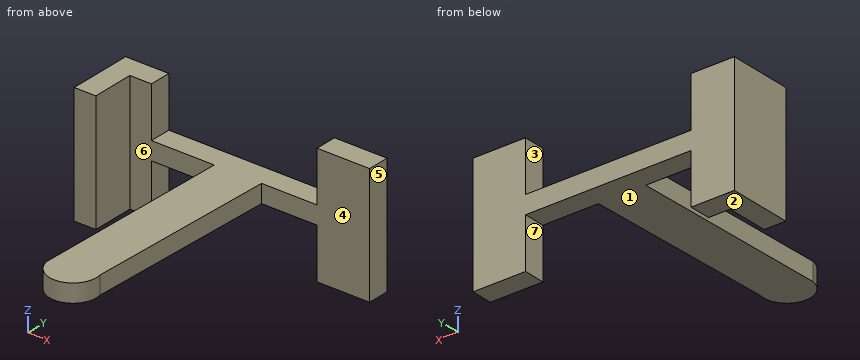
Autodesk Inventor part; units mm, degrees
ref_plane "Work Plane5" through (0, 0, 9.5) normal (0, 0, 1) x (1, 0, 0)
ref_plane "Work Plane4" through (-12.5, 22.5, 0) normal (0, 1, 0) x (1, 0, 0)
ref_plane "YZ Plane" through (0, 0, 0) normal (1, 0, 0) x (0, 1, 0)
ref_plane "Work Plane5" through (0, 0, 9.5) normal (0, 0, 1) x (1, 0, 0)
sketch "Sketch4" plane through (0, 0, 9.5) normal (0, 0, 1) x (1, 0, 0)
  arc A0 (-3.3085, -7.69) -> (3.0707, -6.4871) centre (-0.1029, -7.1736) ccw
  line L0 (3.0707, -6.4871) -> (3.7901, 20.5)
  line L1 (-2.7798, 20.5) -> (-3.3085, -7.69)
  line L2 (-3.8298, 20.5) -> (-2.7798, 20.5)
  line L3 (3.7901, 20.5) -> (4.8401, 20.5)
  line L4 (-11.5, 20.5) -> (-12.5, 20.5)
  line L5 (11.5, 20.5) -> (9.5, 20.5)
  line L6 (-12.5, 20.5) -> (-2.7798, 20.5)
  line L7 (3.7901, 20.5) -> (18.7901, 20.5)
  line L8 (-12.5, 20.5) -> (-12.5, 14.637)
  line L9 (-12.5, 14.637) -> (-12.5, 20.5)
  line L10 (-12.5, 14.637) -> (-14.5, 14.637)
  line L11 (-14.5, 14.637) -> (-14.5, 22.5)
  line L12 (-14.5, 22.5) -> (18.7901, 22.5)
  line L13 (18.7901, 22.5) -> (18.7901, 20.5)
  line L14 (-2.7798, 20.5) -> (3.7901, 20.5)
  point P0 (0, 0)
  point P1 (-0.3189, -10.4133)
  dimension "d34" = 15
  dimension "d36" = 2
  dimension "d52" = 2
extrude "Extrusion7" add sketch "Sketch4" along normal mid plane 2.5 contours L1 L14 L0 A0
extrude "Extrusion8" add sketch "Sketch4" along normal mid plane 17 contours L2 L6 L4 L8 L10 L11 L12 L13 L7 L5 L3 L14
ref_plane "Work Plane4" through (-12.5, 22.5, 0) normal (0, 1, 0) x (1, 0, 0)
sketch "Sketch5" plane through (-12.5, 22.5, 0) normal (0, 1, 0) x (1, 0, 0)
  line L0 (-2, -11.5) -> (27, -11.5)
  line L1 (27, -11.5) -> (27, -7.5)
  line L2 (27, -7.5) -> (-2, -7.5)
  line L3 (-2, -7.5) -> (-2, -11.5)
  line L4 (15.5, -9.5) -> (9.5, -9.5)
  line L5 (-2, -11.5) -> (27, -7.5) construction
  line L6 (27, -11.5) -> (-2, -7.5) construction
  line L7 (0, -1) -> (25, -1)
  line L8 (25, -1) -> (25, -7.5)
  line L9 (25, -7.5) -> (0, -7.5)
  line L10 (0, -7.5) -> (0, -1)
  line L11 (0, -9.5) -> (0, -18)
  line L12 (0, -18) -> (31.2901, -18)
  line L13 (0, -11.5) -> (25, -11.5)
  line L14 (25, -11.5) -> (25, -18)
  line L15 (25, -18) -> (0, -18)
  line L16 (0, -18) -> (0, -11.5)
  point P0 (12.5, 0)
  point P1 (12.5, -9.5)
extrude "Extrusion9" cut sketch "Sketch5" against normal through all contours L0 L14 L12 L11 | L10 L7 L8 L2
sketch "Sketch6" plane through (-14.5, 22.5, 1) normal (0, 1, 0) x (1, 0, 0)
  line L0 (2, -6.5) -> (27, -6.5)
  line L1 (2, 0) -> (4, 0)
  line L2 (4, 0) -> (4, -6.5)
  line L3 (4, -6.5) -> (2, -6.5)
  line L4 (2, -6.5) -> (2, 0)
  line L5 (27, -10.5) -> (2, -10.5)
  line L6 (2, -17) -> (4, -17)
  line L7 (4, -17) -> (4, -10.5)
  line L8 (4, -10.5) -> (2, -10.5)
  line L9 (2, -10.5) -> (2, -17)
  line L10 (27, 0) -> (25, 0)
  line L11 (25, 0) -> (25, -6.5)
  line L12 (25, -6.5) -> (27, -6.5)
  line L13 (27, -6.5) -> (27, 0)
  line L14 (27, -10.5) -> (25, -10.5)
  line L15 (25, -10.5) -> (25, -17)
  line L16 (25, -17) -> (27, -17)
  line L17 (27, -17) -> (27, -10.5)
  point P0 (14.5, 1)
  dimension "d43" = 2
  dimension "d44" = 2
  dimension "d45" = 2
  dimension "d46" = 2
extrude "Extrusion10" add sketch "Sketch6" along normal mid plane 4
sketch "Sketch7" plane through (18.7901, 22.5, 18) normal (0, 1, 0) x (1, 0, 0)
  line L0 (-8.2901, 0) -> (0, 0)
  line L1 (0, 17) -> (5, 17)
  line L2 (5, 17) -> (5, 0)
  line L3 (5, 0) -> (0, 0)
  line L4 (0, 0) -> (0, 17)
  point P0 (-18.7901, 18)
  dimension "d49" = 5
extrude "Extrusion11" cut sketch "Sketch7" against normal through all
sketch "Sketch8" plane through (0, 0, 18) normal (0, 0, 1) x (1, 0, 0)
  line L0 (12.5, 24.5) -> (18.7901, 24.5)
  line L1 (18.7901, 24.5) -> (18.7901, 22.5)
  line L2 (18.7901, 22.5) -> (12.5, 22.5)
  line L3 (12.5, 22.5) -> (12.5, 24.5)
  line L4 (-12.5, 24.5) -> (-14.5, 24.5)
  line L5 (-14.5, 24.5) -> (-14.5, 22.5)
  line L6 (-14.5, 22.5) -> (-12.5, 22.5)
  line L7 (-12.5, 22.5) -> (-12.5, 24.5)
  point P0 (0, 0)
extrude "Extrusion12" add sketch "Sketch8" against normal blind 17
sketch "Sketch9" plane through (-10.5, 22.5, 11.5) normal (0, 1, 0) x (1, 0, 0)
  line L0 (0, 0) -> (0, 4)
  line L1 (21, 0) -> (21, 4)
  line L2 (23, 0) -> (21, 0)
  line L3 (23, 0) -> (23, 4)
  line L4 (21, 4) -> (23, 4)
  line L5 (-2, 4) -> (0, 4)
  line L6 (-2, 0) -> (-2, 4)
  line L7 (0, 0) -> (-2, 0)
  point P0 (10.5, 11.5)
extrude "Extrusion13" add sketch "Sketch9" along normal blind 2
sketch "Sketch10" plane through (-10.5, 20.5, 11.5) normal (0, 0, 1) x (1, 0, 0)
  line L0 (0, 4) -> (21, 4)
  line L1 (21, 4) -> (21, 2)
  line L2 (21, 2) -> (0, 2)
  line L3 (0, 2) -> (0, 4)
  point P0 (10.5, -20.5)
extrude "Extrusion14" add sketch "Sketch10" against normal blind 4
sketch "Sketch12" plane through (0, 0, 18) normal (0, 0, 1) x (1, 0, 0)
  line L0 (18.7901, 24.5) -> (18.7901, 20.5)
  line L1 (-14.5, 24.5) -> (18.7901, 24.5)
  line L2 (18.7901, 24.5) -> (18.7901, 23.5)
  line L3 (18.7901, 23.5) -> (-14.5, 23.5)
  line L4 (-14.5, 23.5) -> (-14.5, 24.5)
  point P0 (0, 0)
  dimension "d59" = 1
extrude "Extrusion15" cut sketch "Sketch12" against normal through all
sketch "Sketch13" plane through (0, 0, 18) normal (0, 0, 1) x (1, 0, 0)
  line L0 (-14.5, 23.5) -> (-15.5, 23.5)
  line L1 (-15.5, 23.5) -> (-15.5, 14.637)
  line L2 (-15.5, 14.637) -> (-14.5, 14.637)
  line L3 (-14.5, 14.637) -> (-14.5, 23.5)
  point P0 (0, 0)
  dimension "d62" = 1
extrude "Extrusion16" add sketch "Sketch13" against normal blind 17
sketch "Sketch15" plane through (10.5, 23.5, 18) normal (0, 1, 0) x (1, 0, 0)
  line L0 (0, 17) -> (3, 17)
  line L1 (3, 17) -> (3, 10.5)
  line L2 (3, 10.5) -> (0, 10.5)
  line L3 (0, 10.5) -> (0, 17)
  line L4 (0, 0) -> (3, 0)
  line L5 (3, 0) -> (3, 6.4739)
  line L6 (3, 6.4739) -> (0, 6.4739)
  line L7 (0, 6.4739) -> (0, 0)
  point P0 (-10.5, 18)
  dimension "d70" = 3
extrude "Extrusion18" cut sketch "Sketch15" against normal up to next
sketch "Sketch16" plane through (-10.5, 23.5, 11.5) normal (0, 1, 0) x (1, 0, 0)
  line L0 (0, 10.5) -> (1, 10.5)
  line L1 (1, 10.5) -> (1, -6.5)
  line L2 (1, -6.5) -> (0, -6.5)
  line L3 (0, -6.5) -> (0, 10.5)
  point P0 (10.5, 11.5)
extrude "Extrusion19" add sketch "Sketch16" against normal blind 3
sketch "Sketch17" plane through (-12.5, 14.637, 18) normal (1, 0, 0) x (0, 0, -1)
  line L0 (17, 5.863) -> (0, 5.863)
  line L1 (0, 0) -> (0, 5.863)
  line L2 (17, 0) -> (0, 0)
  line L3 (17, 5.863) -> (17, 0)
  point P0 (18, -14.637)
extrude "Extrusion20" cut sketch "Sketch17" against normal blind 2
sketch "Sketch18" plane through (-15.5, 14.637, 18) normal (-1, 0, 0) x (0, 0, 1)
  line L0 (0, 5.863) -> (-17, 5.863)
  line L1 (0, 8.863) -> (0, 0)
  line L2 (0, 8.863) -> (-17, 8.863)
  line L3 (-17, 0) -> (-17, 8.863)
  line L4 (0, 0) -> (-17, 0)
  point P0 (-18, -14.637)
extrude "Extrusion21" add sketch "Sketch18" along normal blind 2
sketch "Sketch19" plane through (18.7901, 23.5, 18) normal (0, 1, 0) x (1, 0, 0)
  line L0 (-28.2901, 17) -> (-30.2901, 17)
  line L1 (-30.2901, 17) -> (-30.2901, 10.5)
  line L2 (-30.2901, 10.5) -> (-28.2901, 10.5)
  line L3 (-28.2901, 10.5) -> (-28.2901, 17)
  line L4 (-28.2901, 0) -> (-36.2901, 0)
  line L5 (-28.2901, 6.5) -> (-30.2901, 6.5)
  line L6 (-30.2901, 6.5) -> (-30.2901, 0)
  line L7 (-30.2901, 0) -> (-28.2901, 0)
  line L8 (-28.2901, 0) -> (-28.2901, 6.5)
  line L9 (-5.2901, 17) -> (-7.2901, 17)
  line L10 (-7.2901, 17) -> (-7.2901, 0)
  line L11 (-7.2901, 0) -> (-5.2901, 0)
  line L12 (-5.2901, 0) -> (-5.2901, 17)
  point P0 (-18.7901, 18)
  dimension "d77" = 2
  dimension "d78" = 2
extrude "Extrusion22" cut sketch "Sketch19" against normal up to next contours L3 L2 L1 L0 | L4 L6 L5 L8
extrude "Extrusion23" add sketch "Sketch19" against normal blind 3 contours L12 L11 L10 L9
sketch "Sketch20" plane through (18.7901, 20.5, 1) normal (0, -1, 0) x (1, 0, 0)
  line L0 (-22.0985, 7.25) -> (-15.646, 7.25)
  line L1 (-15.646, 9.75) -> (-22.0985, 9.75)
  line L2 (-7.2901, 17) -> (-7.2901, 10.5261)
  line L3 (-30.2901, 17) -> (-30.2901, 10.5)
  line L4 (-30.2901, 13) -> (-7.2901, 13)
  line L5 (-7.2901, 13) -> (-7.2901, 9.75)
  line L6 (-7.2901, 9.75) -> (-30.2901, 9.75)
  line L7 (-30.2901, 9.75) -> (-30.2901, 13)
  line L8 (-30.2901, 4) -> (-7.2901, 4)
  line L9 (-7.2901, 4) -> (-7.2901, 7.25)
  line L10 (-7.2901, 7.25) -> (-30.2901, 7.25)
  line L11 (-30.2901, 7.25) -> (-30.2901, 4)
  point P0 (-18.7901, -1)
  point P1 (-15.7194, 7.25)
  point P2 (-15.7194, 9.75)
extrude "Extrusion24" cut sketch "Sketch20" against normal through all
sketch "Sketch21" plane through (18.7901, 23.5, 18) normal (0, 1, 0) x (1, 0, 0)
  line L0 (0, 17) -> (0, 0)
  line L1 (-36.2901, 17) -> (0, 17)
  line L2 (0, 17) -> (0, 16.75)
  line L3 (0, 16.75) -> (-36.2901, 16.75)
  line L4 (-36.2901, 16.75) -> (-36.2901, 17)
  line L5 (-36.2901, 0) -> (-36.2901, 17)
  line L6 (0, 0) -> (-36.2901, 0)
  line L7 (-36.2901, 0) -> (-36.2901, 0.25)
  line L8 (-36.2901, 0.25) -> (0, 0.25)
  line L9 (0, 0.25) -> (0, 0)
  point P0 (-18.7901, 18)
  dimension "d85" = 0.25
  dimension "d86" = 0.25
extrude "Extrusion25" cut sketch "Sketch21" against normal through all contours L0 L3 L4 L1 | L0 L6 L5 L8
properties part number "cover sepatu32"
Design review of the part built by this model. Coordinates are the model's own, in mm. Face numbers are marked on the shaded views. A direction names the side the tool comes from. Coordinates: 2 decimals unless noted, no trailing zeros. Order: outer loops, then holes, each group sorted by start corner. A loop starts at its lowest first (then second) coordinate and runs counter-clockwise, first axis right, second up. Notation, with made-up numbers: M 83,8 L 93,8 A19 ccw 93,24 Z; hole C 44,-19.75 d5. An arc over 180 degrees is marked long. Answer as a JSON object with one key per item and string values. Group by question number.
1) Tool access review of the marked faces 1, 2 and 3: name each direction out of +Z, -Z, +X, -X, +Y, -Y from which nothing blocks a thin tool from reaching the whole face with its end or side.
2) Add section A-A, the plane z = 15.5. Write out the cut boundary in (x, y).
3) Add section C-C, the plane y = 0.5. Write out the cut boundary in (x, z), then the cut area to 3 significant figures.
4) Wall thickness on L1, parallel to X at y = 21.5, z = 12; L2, parallel to Y at x = -12, z = 16.5; L3, parallel to Z at x = -1, y = 6: over which ranges is each line inside the solid? List them lowest first.
5) Add section B-B, the plane x = 15.5. Write out the cut boundary in (y, z), then the cut area to 3 significant figures.
6) Mouldability with a two-part tool opening along X and no side actions: class the marked faces 4, 5, 6 and 7 as pulls with the +X half, pulls with the -X half, needs draft (parallel to the pull), parting line crosses it, or undercut.
7) For pin 1 (5 mm diameter, centred on x = -3.5, z = 13.5, fed in from +Y); pin 2 (2 mm diameter, centred on x = 6.5, z = 9, fed in from -Y); pin 3 (8 mm diameter, centred on y = 11.5, z = 14, fed in from +X); pin 4 (5 mm diameter, centred on y = -3, z = 9, fed in from -X), all flat-tipped, find the tip position at first contact; note any pin that passes through.
Computed values:
{
 "1": {"face 1": "-Z, +Y, -Y", "face 2": "-Z, +X, -X, +Y, -Y", "face 3": "+Z, +Y, -Y"},
 "2": {"outline": "M -17.5,14.64 L -14.5,14.64 L -14.5,20.5 L -11.5,20.5 L -11.5,23.5 L -17.5,23.5 Z; M 11.5,20.5 L 18.79,20.5 L 18.79,23.5 L 11.5,23.5 Z"},
 "3": {"outline": "M -3.15,8.25 L 3.26,8.25 L 3.26,10.75 L -3.15,10.75 Z", "area": "16.0 mm^2"},
 "4": {"L1": "x = -17.5 to -11.5, 11.5 to 18.79", "L2": "y = 20.5 to 23.5", "L3": "z = 8.25 to 10.75"},
 "5": {"outline": "M 20.5,1.25 L 23.5,1.25 L 23.5,17.75 L 20.5,17.75 Z", "area": "49.5 mm^2"},
 "6": {"face 4": "needs draft", "face 5": "pulls with the +X half", "face 6": "undercut", "face 7": "undercut"},
 "7": {"pin 1": "passes through", "pin 2": "stops at y = 20.5", "pin 3": "stops at x = 3.61", "pin 4": "stops at x = -3.27"}
}
